Could you check a few things on this model? Use its own coordinates, in mm. Coordinates: 2 decimals unless noted, no trailing zeros. Loops run counter-clockwise (first coordinate to the right, second up) from the corner with the lowest first, then second, coordinate; pieces in that order, holes last. Notation, with made-up numbers: (18, -2) -> (28, -2) arc R15 ccw to (28, 25) -> close; hole circle Ø11 at (-25, 72). An arc over 180 degrees is marked (long way). One line per question, with ' | ' between items.
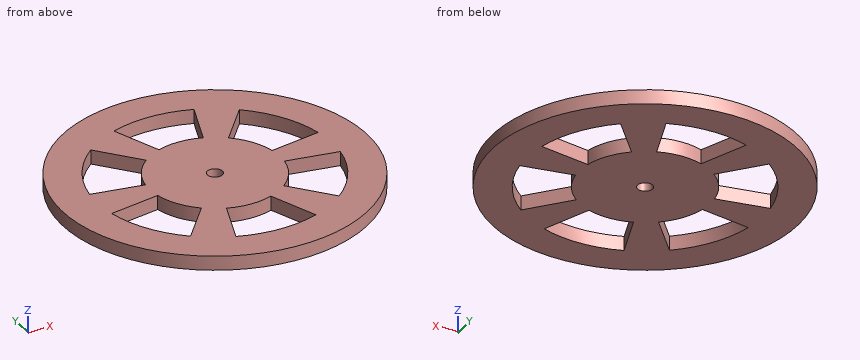
```python
from build123d import *

# Parameters (mm, degrees)
MODEL_R             = 30
MODEL_R_2           = 1.5
BOSS_EXTRUDE1_DEPTH = 2.8


with BuildPart() as part:
    # Model → Boss-Extrude1 (new body)
    with BuildSketch(Plane.XY):
        with Locations((183.021792723, 1.638749849)):
            Circle(MODEL_R)
        with Locations((183.021792723, 1.638749849)):
            Circle(MODEL_R_2, mode=Mode.SUBTRACT)
        with BuildLine():
            Line((160.184310638, 5.594924102), (170.361966665, 3.831832156))
            ThreePointArc((170.361966665, 3.831832156), (171.89553669, 8.064264032), (174.794965696, 11.507899908))
            Line((174.794965696, 11.507899908), (168.18114531, 19.442038508))
            ThreePointArc((168.18114531, 19.442038508), (162.950768709, 13.229948999), (160.184310638, 5.594924102))
        make_face(mode=Mode.SUBTRACT)
        with BuildLine():
            Line((160.183368767, -2.31198349), (170.361444544, -0.551316319))
            ThreePointArc((170.361444544, -0.551316319), (171.894006192, -4.784113433), (174.792614703, -8.228439971))
            Line((174.792614703, -8.228439971), (168.176904275, -16.161002669))
            ThreePointArc((168.176904275, -16.161002669), (162.948007791, -9.947667252), (160.183368767, -2.31198349))
        make_face(mode=Mode.SUBTRACT)
        with BuildLine():
            Line((175.02401618, -20.115272149), (178.588271571, -10.420466378))
            ThreePointArc((178.588271571, -10.420466378), (183.020262224, -11.209627616), (187.452440761, -10.421522278))
            Line((187.452440761, -10.421522278), (191.01438636, -20.117176922))
            ThreePointArc((191.01438636, -20.117176922), (183.019031805, -21.538866402), (175.02401618, -20.115272149))
        make_face(mode=Mode.SUBTRACT)
        with BuildLine():
            Line((197.862440136, -16.16453881), (191.248619749, -8.23040021))
            ThreePointArc((191.248619749, -8.23040021), (194.148048755, -4.786764334), (195.68161878, -0.554332458))
            Line((195.68161878, -0.554332458), (205.859274808, -2.317424405))
            ThreePointArc((205.859274808, -2.317424405), (203.092816736, -9.952449302), (197.862440136, -16.16453881))
        make_face(mode=Mode.SUBTRACT)
        with BuildLine():
            Line((205.860216679, 5.589483188), (195.682140901, 3.828816016))
            ThreePointArc((195.682140901, 3.828816016), (194.149579254, 8.06161313), (191.250970742, 11.505939668))
            Line((191.250970742, 11.505939668), (197.86668117, 19.438502366))
            ThreePointArc((197.86668117, 19.438502366), (203.095577654, 13.225166949), (205.860216679, 5.589483188))
        make_face(mode=Mode.SUBTRACT)
        with BuildLine():
            Line((191.019569265, 23.392771846), (187.455313874, 13.697966076))
            ThreePointArc((187.455313874, 13.697966076), (183.023323222, 14.487127313), (178.591144685, 13.699021976))
            Line((178.591144685, 13.699021976), (175.029199085, 23.39467662))
            ThreePointArc((175.029199085, 23.39467662), (183.024553641, 24.8163661), (191.019569265, 23.392771846))
        make_face(mode=Mode.SUBTRACT)
    extrude(amount=BOSS_EXTRUDE1_DEPTH)


solid = part.part
```
Q1. Imagine slicing it at A-A on y = -12. Write out the boundary of the cut face in (x, z), plus the area to 3 significant figures.
Values follow:
outline: (156.3, 0) -> (164.28, 0) -> (164.28, 2.8) -> (156.3, 2.8) -> close; (171.65, 0) -> (178.01, 0) -> (178.01, 2.8) -> (171.65, 2.8) -> close; (188.03, 0) -> (194.39, 0) -> (194.39, 2.8) -> (188.03, 2.8) -> close; (201.76, 0) -> (209.74, 0) -> (209.74, 2.8) -> (201.76, 2.8) -> close | area: 80.3 mm2
Q2. Imagine slicing it at D-D on y = -6. Write out the boundary of the cut face in (x, z), plus the area to 3 significant figures.
Values follow:
outline: (154.01, 0) -> (161.14, 0) -> (161.14, 2.8) -> (154.01, 2.8) -> close; (172.69, 0) -> (193.35, 0) -> (193.35, 2.8) -> (172.69, 2.8) -> close; (204.9, 0) -> (212.03, 0) -> (212.03, 2.8) -> (204.9, 2.8) -> close | area: 97.8 mm2
Q3. For pin 1 (3 mm diameter, centred on x = 169, y = -3.5, fed in from +Z); pin 2 (4 mm diameter, centred on x = 162, y = 1, fed in from -Z); pin 3 (1.5 mm diameter, centred on y = 15.5, z = 1, fed in from +X), each with a flat end and sliding along its axis, tell me the tip position at first contact or that it passes through.
Values follow:
pin 1: passes through | pin 2: stops at z = 0 | pin 3: stops at x = 210.01
Q4. Imagine slicing it at B-B on x = 165. Write out the boundary of the cut face in (y, z).
Values follow:
outline: (-22.34, 0) -> (-12.94, 0) -> (-12.94, 2.8) -> (-22.34, 2.8) -> close; (-1.48, 0) -> (4.76, 0) -> (4.76, 2.8) -> (-1.48, 2.8) -> close; (16.21, 0) -> (25.62, 0) -> (25.62, 2.8) -> (16.21, 2.8) -> close
Q5. Imagine slicing it at C-C on z = 2.05. Write out the boundary of the cut face in (x, y).
Values follow:
outline: circle Ø60 at (183.02, 1.64); hole (160.18, -2.31) arc R23.18 ccw to (168.18, -16.16) -> (174.79, -8.23) arc R12.85 cw to (170.36, -0.55) -> close; hole (160.18, 5.59) -> (170.36, 3.83) arc R12.85 cw to (174.79, 11.51) -> (168.18, 19.44) arc R23.18 ccw to start; hole (175.02, -20.12) arc R23.18 ccw to (191.01, -20.12) -> (187.45, -10.42) arc R12.85 cw to (178.59, -10.42) -> close; hole (175.03, 23.39) -> (178.59, 13.7) arc R12.85 cw to (187.46, 13.7) -> (191.02, 23.39) arc R23.18 ccw to start; hole circle Ø3 at (183.02, 1.64); hole (191.25, -8.23) -> (197.86, -16.16) arc R23.18 ccw to (205.86, -2.32) -> (195.68, -0.55) arc R12.85 cw to start; hole (191.25, 11.51) arc R12.85 cw to (195.68, 3.83) -> (205.86, 5.59) arc R23.18 ccw to (197.87, 19.44) -> close
Q6. Please list where these lines run through material, in increasing order: L1, parallel to Y at x = 173.5, z = 1.6; L2, parallel to Y at x = 194.5, z = 1.2; L3, parallel to X at y = 7.5, z = 0.8. Write a range as [from, to].
Values follow:
L1: y = [-26.81, -9.78], [-6.99, 10.27], [13.06, 30.09] | L2: y = [-26.08, -12.13], [-4.13, 7.41], [15.4, 29.36] | L3: x = [153.6, 160.6], [171.59, 194.46], [205.45, 212.44]
